```python
from build123d import *

# Parameters (mm, degrees)
SKETCH2_R           = 144.505
BOSS_EXTRUDE1_DEPTH = 7.5
SKETCH3_R           = 40
SKETCH3_R_2         = 15
CUT_EXTRUDE1_DEPTH  = 16


with BuildPart() as part:
    # Sketch2 → Boss-Extrude1 (new body, symmetric)
    with BuildSketch(Plane.XY):
        Circle(SKETCH2_R)
    extrude(amount=BOSS_EXTRUDE1_DEPTH, both=True)

    # Sketch3 → Cut-Extrude1 (cut, through all)
    with BuildSketch(Plane.XY.offset(7.5)):
        Circle(SKETCH3_R)
        with Locations((0, 75)):
            Circle(SKETCH3_R_2)
        with Locations((44.083893922, 60.676274578)):
            Circle(SKETCH3_R_2)
        with Locations((71.329238722, 23.176274578)):
            Circle(SKETCH3_R_2)
        with Locations((71.329238722, -23.176274578)):
            Circle(SKETCH3_R_2)
        with Locations((44.083893922, -60.676274578)):
            Circle(SKETCH3_R_2)
        with Locations((0, -75)):
            Circle(SKETCH3_R_2)
        with Locations((-44.083893922, -60.676274578)):
            Circle(SKETCH3_R_2)
        with Locations((-71.329238722, -23.176274578)):
            Circle(SKETCH3_R_2)
        with Locations((-71.329238722, 23.176274578)):
            Circle(SKETCH3_R_2)
        with Locations((-44.083893922, 60.676274578)):
            Circle(SKETCH3_R_2)
    extrude(amount=-CUT_EXTRUDE1_DEPTH, mode=Mode.SUBTRACT)


solid = part.part
```
Build history of the part. All positions in model axes, mm. Give positions to 0.01 mm unless a question says otherwise; leave off trailing zeros. Loops run counter-clockwise (first coordinate to the right, second up) from the corner with the lowest first, then second, coordinate; pieces in that order, holes last.
Item 1: Flat gauge pins, fed straight in: pin 1 (1 mm diameter, centred on x = -109, z = -3, fed in from +Y); pin 2 (8 mm diameter, centred on y = 100.5, z = 2, fed in from -X); pin 3 (3 mm diameter, centred on y = 45, z = -1.5, fed in from -X). Where does each tip first touch, or does it go through?
Answers follow:
pin 1: stops at y = 95.44
pin 2: stops at x = -107.56
pin 3: stops at x = -137.8
Item 2: Slice it at B-B, the plane x = 0. List the corners of the cut face in (y, z) (3 decimals).
Answers follow:
outline: (-144.505, -7.5) - (-90, -7.5) - (-90, 7.5) - (-144.505, 7.5) - close; (-60, -7.5) - (-40, -7.5) - (-40, 7.5) - (-60, 7.5) - close; (40, -7.5) - (60, -7.5) - (60, 7.5) - (40, 7.5) - close; (90, -7.5) - (144.505, -7.5) - (144.505, 7.5) - (90, 7.5) - close
Item 3: Drill centre lines: line 1 (Y direction, x = 45, z = 5.5); line 2 (X direction, y = -28, z = 2.5); line 3 (X direction, y = 23.5, z = -2.25). Where is each one in solid material? Low to high.
Answers follow:
line 1: y = -137.32 to -75.65, -45.7 to 45.7, 75.65 to 137.32
line 2: x = -141.77 to -85.53, -57.13 to -28.57, 28.57 to 57.13, 85.53 to 141.77
line 3: x = -142.58 to -86.33, -56.33 to -32.37, 32.37 to 56.33, 86.33 to 142.58
Item 4: Slice it at D-D, the plane y = 104. List the corners of the cut face in (x, z), and give its area (3 significant figures).
Answers follow:
outline: (-100.33, -7.5) - (100.33, -7.5) - (100.33, 7.5) - (-100.33, 7.5) - close
area: 3,010 mm2
Item 5: Pull direction X, two halves, no side cores. Call faces 1 (the face through (30, -30, 7.5)), 2 (the face through (-36.02, 73.324, 0.105)), 3 (the face through (-114.674, -87.929, 0.105)): released by +X, released by -X, zero draft, split by the parting line, or undercut.
Answers follow:
face 1: zero draft
face 2: undercut
face 3: split by the parting line
Item 6: Slice it at A-A, the plane y = 0. List the corners of the cut face in (x, z) (3 decimals).
Answers follow:
outline: (-144.505, -7.5) - (-40, -7.5) - (-40, 7.5) - (-144.505, 7.5) - close; (40, -7.5) - (144.505, -7.5) - (144.505, 7.5) - (40, 7.5) - close
Item 7: Slice it at C-C, the plane z = -3. Give the number of separate pieces and of enclosed holes in the cut face, and give its area (3 significant figures).
Answers follow:
separate pieces: 1
enclosed holes: 11
area: 53,500 mm2
